```python
from build123d import *

# Parameters (mm, degrees)
F1_DEPTH = 40
F2_R     = 10
F3_DEPTH = 5
F6_DEPTH = 15
F7_SIZE  = 2.5


with BuildPart() as f1:
    # F0 (on Front) → F1 (new body)
    with BuildSketch(Plane.XZ):
        with BuildLine():
            Line((-20, 0), (-20, -7.889866919))
            ThreePointArc((-20, -7.889866919), (-15.2027957955, -15.2027957955), (-7.889866919, -20))
            Line((-7.889866919, -20), (0, -20))
            Line((0, -20), (0, -10))
            ThreePointArc((0, -10), (-7.0710678119, -7.0710678119), (-10, 0))
            Line((-10, 0), (-20, 0))
        make_face()
        with BuildLine():
            ThreePointArc((7.889866919, -20), (15.2027957955, -15.2027957955), (20, -7.889866919))
            Line((20, -7.889866919), (20, 0))
            Line((20, 0), (10, 0))
            ThreePointArc((10, 0), (7.0710678119, -7.0710678119), (0, -10))
            Line((0, -10), (0, -20))
            Line((0, -20), (7.889866919, -20))
        make_face()
        with BuildLine():
            Line((20, 0), (20, 7.889866919))
            ThreePointArc((20, 7.889866919), (0, 21.5), (-20, 7.889866919))
            Line((-20, 7.889866919), (-20, 0))
            Line((-20, 0), (-10, 0))
            ThreePointArc((-10, 0), (0, 10), (10, 0))
            Line((10, 0), (20, 0))
        make_face()
    extrude(amount=F1_DEPTH)

    # F2 (on face) → F3 (join)
    with BuildSketch(Plane(origin=(0, 0, 0), x_dir=(-1, 0, 0), z_dir=(0, 1, 0))):
        with BuildLine():
            ThreePointArc((20, 7.889866919), (0, 21.5), (-20, 7.889866919))
            Line((-20, 7.889866919), (-20, -7.889866919))
            ThreePointArc((-20, -7.889866919), (-15.2027957955, -15.2027957955), (-7.889866919, -20))
            Line((-7.889866919, -20), (7.889866919, -20))
            ThreePointArc((7.889866919, -20), (15.2027957955, -15.2027957955), (20, -7.889866919))
            Line((20, -7.889866919), (20, 7.889866919))
        make_face()
        Circle(F2_R, mode=Mode.SUBTRACT)
        Circle(F2_R)
    extrude(amount=F3_DEPTH)

    # F5 (on offset) → F6 (cut)
    with BuildSketch(Plane.XY.offset(21.5)):
        with BuildLine():
            ThreePointArc((0, -17), (-2.1213203436, -22.1213203436), (3, -20))
            ThreePointArc((3, -20), (2.1213203436, -17.8786796564), (0, -17))
        make_face()
    extrude(amount=-F6_DEPTH, mode=Mode.SUBTRACT)

    # F7
    f7_edges = [f1.edges().sort_by_distance(p)[0] for p in [
        (10, -40, 0),
    ]]
    chamfer(f7_edges, length=F7_SIZE)


solid = f1.part
```
The listing builds one solid part. Answer for the finished solid, in the listing's coordinates (mm). Coordinates: 2 decimals unless noted, no trailing zeros. Loops run counter-clockwise (first coordinate to the right, second up) from the corner with the lowest first, then second, coordinate; pieces in that order, holes last. Notation, with made-up numbers: (16, 8) -> (65, 8) arc R28 cw to (65, 28) -> close; hole circle Ø4 at (23.25, -28). An arc over 180 degrees is marked (long way). Return JSON: item names as keys, results as strings. Group by question number.
(1) Given pin 1 Ø1.5 at (y, z) = (-32.5, 10.5) entering from -X; pin 2 Ø5 at (x, y) = (-13.5, -17.5) entering from +Z; pin 3 Ø6 at (x, z) = (-3.5, 2) entering from -Y, each flat-ended and moving along its own axis, determine where each tip first touches the part or whether it passes through.
(2) Find the intervals of material crossed by probe 1 along X at (y, z) = (-20, 16); probe 2 along X at (y, z) = (-20, 18); probe 3 along Z at (x, y) = (-6, -32), in increasing order. Write a range as from..to.
(3) A cutting plane is placed at B-B on z = 14. Write down the section's boundary in (x, y).
(4) A cutting plane is placed at A-A on y = -25.5. Write down the section's boundary in (x, z), and give its area (3 significant figures).
(5) Determine the mould class of faces 1 (the cylindrical face through (15.29, -17.815, -15.115)), 2 (the flat face through (0, 0, 0)), 3 (the flat face through (-20, -18, 0)) for opening direction Z: released by +Z, released by -Z, zero draft, split by the parting line, or undercut.
The answers:
{
 "1": {"pin 1": "stops at x = -19.16", "pin 2": "stops at z = 18.47", "pin 3": "stops at y = 0"},
 "2": {"probe 1": "x = -14.36..-3, 3..14.36", "probe 2": "x = -11.76..-3, 3..11.76", "probe 3": "z = -20..-8, 8..20.65"},
 "3": {"outline": "(-16.32, -40) -> (16.32, -40) -> (16.32, 5) -> (-16.32, 5) -> close; hole circle Ø6 at (0, -20)"},
 "4": {"outline": "(-20, -7.89) arc R21.5 ccw to (-7.89, -20) -> (7.89, -20) arc R21.5 ccw to (20, -7.89) -> (20, 7.89) arc R21.5 ccw to (-20, 7.89) -> close; hole circle Ø20 at (0, 0)", "area": "1,090 mm^2"},
 "5": {"face 1": "released by -Z", "face 2": "undercut", "face 3": "zero draft"}
}
